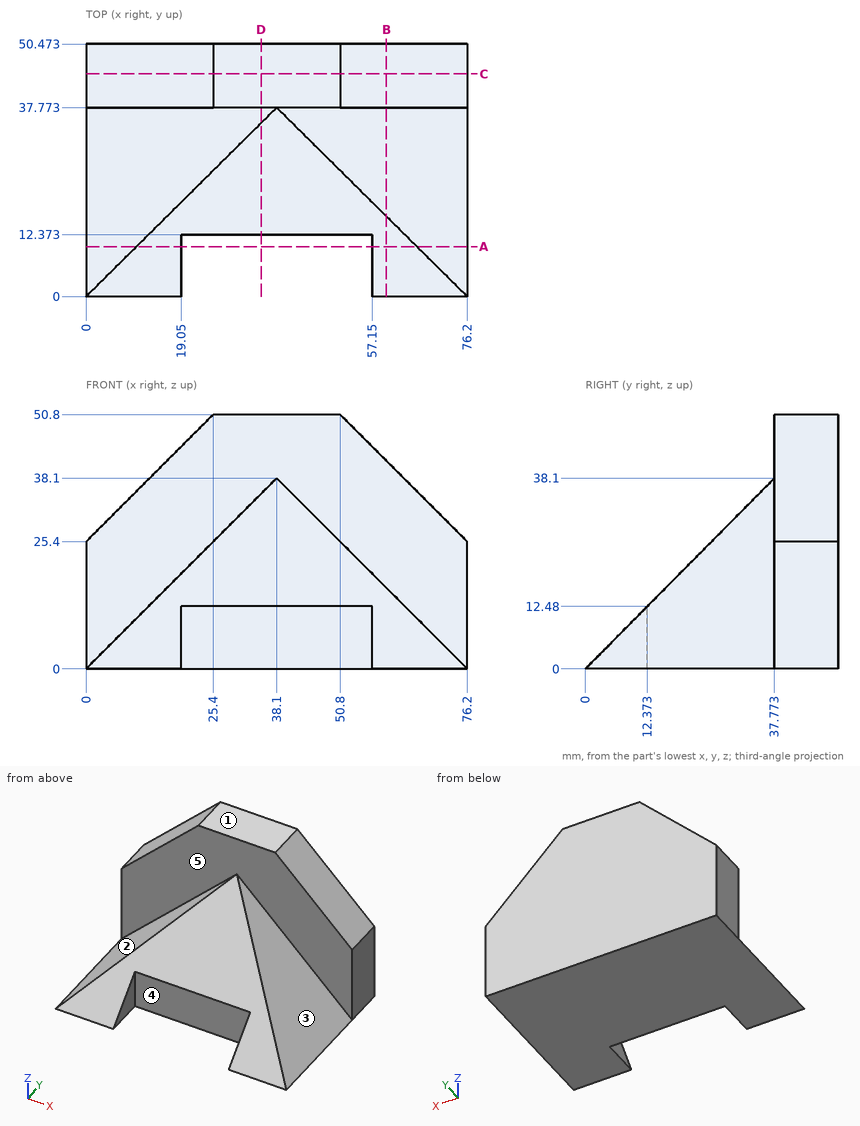
Geometry check sheet. Reference: drawing and pictorial views, mm from the part's lowest x, y, z. A direction names the side the tool comes from. Round coordinates to 2 decimals unless told otherwise and drop trailing zeros. Loops run counter-clockwise (first coordinate to the right, second up) from the corner with the lowest first, then second, coordinate; pieces in that order, holes last. Notation, with made-up numbers: (0, 65) - (21, 65) arc R5 cw to (21, 69) - close; hole circle Ø9 at (22.5, 17.25). An arc over 180 degrees is marked (long way). Write item = value, one per line. Start each with the question number.
Q1. Release check for a two-part mould opening along X. For the marked faces 3, 4 and 5 record: pulls with the +X half, pulls with the -X half, needs draft (parallel to the pull), parting line crosses it, or undercut.
Q2. Access from +Z, -Z, +X, -X, +Y, -Y to the whole of each face (thin tool, end or side, straight path). Record for the marked faces 1 and 2.
Q3. Thickness scan on L1, parallel to Y at x = 18.5, z = 37; L2, parallel to X at y = 7.5, z = 3; L3, parallel to Y at x = 35, z = 10.5. Record the ranges inside material, lowest first.
Q4. Section check D-D (x = 35). Record the boundary of the cut face in (y, z), plus the area to 3 significant figures.
Q5. Section check C-C (y = 44.5). Record the boundary of the cut face in (x, z), plus the area to 3 significant figures.
Q6. Depth check by flat-ended pin: P1, Ø1, axis at x = 57, z = 18, coming from the -Y side; P2, Ø3.5, axis at y = 8.5, z = 6, coming from the +X side; P3, Ø4, axis at x = 21.5, y = 20.5, coming from the +Z side. Enter the tip coordinate at first touch or a pass-through.
Q7. Section check A-A (y = 10). Record the boundary of the cut face in (x, z).
Q8. Section check B-B (x = 60). Record the boundary of the cut face in (y, z), plus the area to 3 significant figures.
Derived:
q1.face_3 = pulls with the +X half
q1.face_4 = undercut
q1.face_5 = needs draft
q2.face_1 = +Z, +X, -X, +Y, -Y
q2.face_2 = +Z, -X, -Y
q3.L1 = 37.77 to 50.47
q3.L2 = 3 to 19.05, 57.15 to 73.2
q3.L3 = 12.37 to 50.47
q4.outline = (12.37, 0) - (50.47, 0) - (50.47, 50.8) - (37.77, 50.8) - (37.77, 35) - (34.7, 35) - (12.37, 12.48) - close
q4.area = 1,280 mm^2
q5.outline = (0, 0) - (76.2, 0) - (76.2, 25.4) - (50.8, 50.8) - (25.4, 50.8) - (0, 25.4) - close
q5.area = 3,230 mm^2
q6.P1 = 17.35
q6.P2 = 71.95
q6.P3 = 22.45
q7.outline = (0, 0) - (19.05, 0) - (19.05, 10.09) - (10.09, 10.09) - close; (57.15, 0) - (76.2, 0) - (66.11, 10.09) - (57.15, 10.09) - close
q8.outline = (0, 0) - (50.47, 0) - (50.47, 41.6) - (37.77, 41.6) - (37.77, 16.2) - (16.06, 16.2) - close
q8.area = 1,010 mm^2
